```python
from build123d import *

# Parameters (mm, degrees)
F1_DEPTH = 500
F3_DEPTH = 25.4
F4_W     = 400
F4_H     = 200
F5_DEPTH = 474.601


# Not quite as in the source:
# - a feature names something its author has since deleted; it is built from what else it names


with BuildPart() as f1:
    # F0 (on Front) → F1 (new body)
    with BuildSketch(Plane.XZ):
        Polygon((350, -350), (350, 350), (-350, 350), (-350, -350), (-150, -350), (-150, -150), (150, -150), (150, -350), align=None)
    extrude(amount=F1_DEPTH)

    # F3 (cut): a face of the model
    f3_faces = [f1.faces().sort_by_distance(p)[0] for p in [
        (0, 0, 34.8837209302),
    ]]
    extrude(f3_faces, amount=-F3_DEPTH, mode=Mode.SUBTRACT)

    # F4 (on face) → F5 (cut, through all)
    with BuildSketch(Plane.XZ.offset(500)):
        Rectangle(F4_W, F4_H)
    extrude(amount=-F5_DEPTH, mode=Mode.SUBTRACT)


solid = f1.part
```
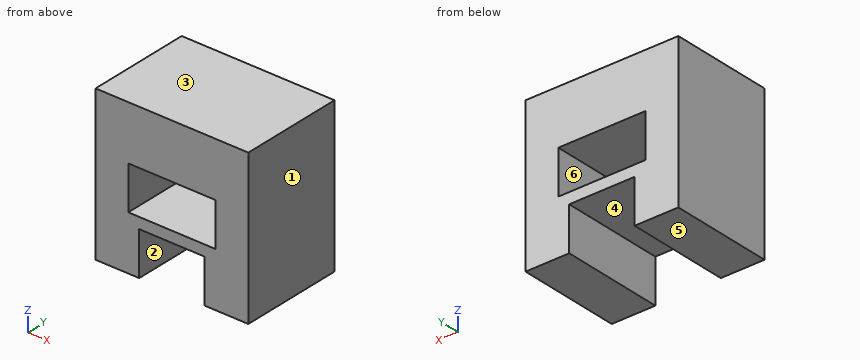
Can you work these out from the model? Positions are in its coordinate system, mm. Face numbers are marked on the shaded views. A direction names the side the tool comes from. Give positions to 0.01 mm unless a question says otherwise; leave off trailing zeros. Order: outer loops, then holes, each group sorted by start corner. A loop starts at its lowest first (then second) coordinate and runs counter-clockwise, first axis right, second up. Notation, with made-up numbers: M 55.5,82.25 L 79.5,82.25 A12 cw 79.5,97.25 Z; hole C 30,57.5 d1. An arc over 180 degrees is marked long. Write item = value, one per line. Start each with the question number.
Q1. For the marked faces 4, 5 and 6, which set-ups out of +Z, -Z, +X, -X, +Y, -Y let a thin tool reach every point of the face, with its end or its side?
Q2. Suppose I cut it at A-A (z = -227). Write out the boundary of the cut face in (x, y).
Q3. We'd pull the mould along X, two halves only. Please class the marked faces 1, 2 and 3: pulls with the +X half, pulls with the -X half, needs draft (parallel to the pull), parting line crosses it, or undercut.
Q4. Suppose I cut it at B-B (x = -82). Write out the boundary of the cut face in (y, z).
Q5. I need wall thicknesses on probe 1 along Z at (x, y) = (64, -238); probe 2 along X at (y, z) = (-340, -308); probe 3 along X at (y, z) = (-290, 93). Which ranges of each line are inside material? Lowest first, please. Write a range as [from, to].
Q6. Suppose I cut it at C-C (y = -442). Write out the boundary of the cut face in (x, z), plus the area to 3 significant figures.
Check result:
q1.face_4 = -Z, +Y, -Y
q1.face_5 = -Z, +X, -X, +Y, -Y
q1.face_6 = +Y, -Y
q2.outline = M -350,-500 L -150,-500 L -150,-25.4 L -350,-25.4 Z; M 150,-500 L 350,-500 L 350,-25.4 L 150,-25.4 Z
q3.face_1 = pulls with the +X half
q3.face_2 = undercut
q3.face_3 = needs draft
q4.outline = M -500,-150 L -25.4,-150 L -25.4,-100 L -500,-100 Z; M -500,100 L -25.4,100 L -25.4,350 L -500,350 Z
q5.probe_1 = [-150, -100], [100, 350]
q5.probe_2 = [-350, -150], [150, 350]
q5.probe_3 = [-350, -200], [200, 350]
q6.outline = M -350,-350 L -150,-350 L -150,-150 L 150,-150 L 150,-350 L 350,-350 L 350,350 L -350,350 Z; hole M -200,-100 L 200,-100 L 200,100 L -200,100 Z
q6.area = 350,000 mm2
